```python
from build123d import *

# Parameters (mm, degrees)
SKETCH1_R               = 1.5
BOSS_EXTRUDE1_DEPTH     = 10
CUT_EXTRUDE1_DEPTH      = 37
CUT_EXTRUDE1_DEPTH_BACK = 24
SKETCH2_R               = 5
CUT_EXTRUDE2_DEPTH      = 27
CUT_EXTRUDE2_DEPTH_BACK = 19
SKETCH3_W               = 102.676723454
SKETCH3_H               = 43.006638415


with BuildPart() as part:
    # Sketch1 → Boss-Extrude1 (new body)
    with BuildSketch(Plane.XY):
        with BuildLine():
            Line((-20, -76.707766284), (-20, -58.504148974))
            Line((-20, -58.504148974), (-120, -58.504148974))
            Line((-120, -58.504148974), (-120, -33.504148974))
            Line((-120, -33.504148974), (-20, -34.707766284))
            Line((-20, -34.707766284), (20, -34.707766284))
            Line((20, -34.707766284), (20, -76.707766284))
            ThreePointArc((20, -76.707766284), (0, -96.707766284), (-20, -76.707766284))
        make_face()
        with Locations((0, -44.707766284)):
            Circle(SKETCH1_R, mode=Mode.SUBTRACT)
        with Locations((-100, -43.745596757)):
            Circle(SKETCH1_R, mode=Mode.SUBTRACT)
    extrude(amount=BOSS_EXTRUDE1_DEPTH)

    # Sketch2 → Cut-Extrude1 (cut, two sides: drawn at the far end of the back side and taken through both)
    with BuildSketch(Plane.XY.offset(10).offset(-CUT_EXTRUDE1_DEPTH_BACK)):
        with Locations((0, -74.90788056)):
            Circle(SKETCH2_R)
    extrude(amount=CUT_EXTRUDE1_DEPTH + CUT_EXTRUDE1_DEPTH_BACK, mode=Mode.SUBTRACT)

    # Sketch3 → Cut-Extrude2 (cut, two sides: drawn at the far end of the back side and taken through both)
    with BuildSketch(Plane.XY.offset(-CUT_EXTRUDE2_DEPTH_BACK)):
        with Locations((-71.338361727, -50.195990653)):
            Rectangle(SKETCH3_W, SKETCH3_H)
    extrude(amount=CUT_EXTRUDE2_DEPTH + CUT_EXTRUDE2_DEPTH_BACK, mode=Mode.SUBTRACT)


solid = part.part
```
Check sheet for the modelled part. Datum: model origin and axes. Units: mm. Coordinates: 2 decimals unless noted, no trailing zeros. Order: outer loops, then holes, each group sorted by start corner. A loop starts at its lowest first (then second) coordinate and runs counter-clockwise, first axis right, second up. Notation, with made-up numbers: M 40,-14 L 76,-14 A35 cw 76,24 Z; hole C 44,24.25 d2. An arc over 180 degrees is marked long. Write each question's results on one line, items separated by ' | '. Start each with the question number.
1. Cross-section at A-A on x = 0. Record the cut outline in (y, z).
2. Material ranges on probe 1 along Y at (x, z) = (0, 2); probe 2 along X at (y, z) = (-75, 2); probe 3 along X at (y, z) = (-44.5, 1.5), recorded low to high.
3. Cross-section at C-C on y = -92.5. Record the cut outline in (x, z).
4. Cross-section at D-D on x = -16. Record the cut outline in (y, z), and give its area (3 significant figures).
5. Cross-section at B-B on z = 3. Record the cut outline in (x, y).
6. Go/stop test with flat-tipped pins: P1, Ø1.5, axis at x = 8, z = 1, coming from the -Y side; P2, Ø4, axis at x = -3, z = 5.5, coming from the -Y side; P3, Ø1, axis at y = -89.5, z = 6, coming from the +X side. Record where each tip stops, or that it passes through.
7. Mould release check, pull along Y, two halves, no side actions. Record for faces 1 (the face through (-1.08, -79.79, 4.93)), 2 (the face through (0, -34.708, 5)), 3 (the face through (-0.33, -46.17, 4.93)), 4 (the face through (20, -55, 5)): +Y half, -Y half, draft (parallel to the pull), parting line (faces both ways), or undercut.
Checks:
1) outline: M -96.71,0 L -79.91,0 L -79.91,10 L -96.71,10 Z; M -69.91,0 L -46.21,0 L -46.21,10 L -69.91,10 Z; M -43.21,0 L -34.71,0 L -34.71,10 L -43.21,10 Z
2) probe 1: y = -96.71 to -79.91, -69.91 to -46.21, -43.21 to -34.71 | probe 2: x = -20 to -5, 5 to 20 | probe 3: x = -20 to -1.49, 1.49 to 20
3) outline: M -12.27,0 L 12.27,0 L 12.27,10 L -12.27,10 Z
4) outline: M -88.71,0 L -34.71,0 L -34.71,10 L -88.71,10 Z | area: 540 mm²
5) outline: M -20,-76.71 A20 ccw 20,-76.71 L 20,-34.71 L -20,-34.71 Z; hole C 0,-74.91 d10; hole C 0,-44.71 d3
6) P1: stops at y = -95.35 | P2: stops at y = -96.68 | P3: stops at x = 15.78
7) face 1: undercut | face 2: +Y half | face 3: undercut | face 4: draft
